```python
from build123d import *

# Parameters (mm, degrees)
SKETCH1_W           = 100
SKETCH1_H           = 100
BASE_DEPTH          = 10
SKETCH2_R           = 10.5
LOAD_CELL_CUT_DEPTH = 1
CUT_EXTRUDE1_REACH  = 12
SKETCH15_R          = 3
SKETCH21_R          = 2.5
CUT_EXTRUDE2_DEPTH  = 10
SKETCH22_R          = 4
CUT_EXTRUDE3_DEPTH  = 11


with BuildPart() as part:
    # Sketch1 → base (new body)
    with BuildSketch(Plane(origin=(0, 0, 0), x_dir=(1, 0, 0), z_dir=(0, 1, 0))):
        Rectangle(SKETCH1_W, SKETCH1_H)
    extrude(amount=BASE_DEPTH)

    # Sketch2 → load cell cut (cut)
    with BuildSketch(Plane(origin=(0, 10, 0), x_dir=(1, 0, 0), z_dir=(0, 1, 0))):
        Circle(SKETCH2_R)
    extrude(amount=-LOAD_CELL_CUT_DEPTH, mode=Mode.SUBTRACT)

    # Sketch15 → Cut-Extrude1 (cut, up to next)
    with BuildSketch(Plane(origin=(0, 0, 0), x_dir=(-1, 0, 0), z_dir=(0, -1, 0)), mode=Mode.PRIVATE) as cut_extrude1_sk1:
        with Locations((40, -40)):
            Circle(SKETCH15_R)
    cut_extrude1_tool1 = extrude(cut_extrude1_sk1.sketch, amount=-CUT_EXTRUDE1_REACH, mode=Mode.PRIVATE) & part.part
    add(cut_extrude1_tool1.solids().sort_by_distance((-40, 0, 40))[0], mode=Mode.SUBTRACT)
    # Sketch15 → Cut-Extrude1 (cut, up to next)
    with BuildSketch(Plane(origin=(0, 0, 0), x_dir=(-1, 0, 0), z_dir=(0, -1, 0)), mode=Mode.PRIVATE) as cut_extrude1_sk2:
        with Locations((-40, -40)):
            Circle(SKETCH15_R)
    cut_extrude1_tool2 = extrude(cut_extrude1_sk2.sketch, amount=-CUT_EXTRUDE1_REACH, mode=Mode.PRIVATE) & part.part
    add(cut_extrude1_tool2.solids().sort_by_distance((40, 0, 40))[0], mode=Mode.SUBTRACT)
    # Sketch15 → Cut-Extrude1 (cut, up to next)
    with BuildSketch(Plane(origin=(0, 0, 0), x_dir=(-1, 0, 0), z_dir=(0, -1, 0)), mode=Mode.PRIVATE) as cut_extrude1_sk3:
        with Locations((40, 40)):
            Circle(SKETCH15_R)
    cut_extrude1_tool3 = extrude(cut_extrude1_sk3.sketch, amount=-CUT_EXTRUDE1_REACH, mode=Mode.PRIVATE) & part.part
    add(cut_extrude1_tool3.solids().sort_by_distance((-40, 0, -40))[0], mode=Mode.SUBTRACT)
    # Sketch15 → Cut-Extrude1 (cut, up to next)
    with BuildSketch(Plane(origin=(0, 0, 0), x_dir=(-1, 0, 0), z_dir=(0, -1, 0)), mode=Mode.PRIVATE) as cut_extrude1_sk4:
        with Locations((-40, 40)):
            Circle(SKETCH15_R)
    cut_extrude1_tool4 = extrude(cut_extrude1_sk4.sketch, amount=-CUT_EXTRUDE1_REACH, mode=Mode.PRIVATE) & part.part
    add(cut_extrude1_tool4.solids().sort_by_distance((40, 0, -40))[0], mode=Mode.SUBTRACT)

    # Sketch21 → Cut-Extrude2 (cut)
    with BuildSketch(Plane(origin=(0, 0, -50), x_dir=(-1, 0, 0), z_dir=(0, 0, -1))):
        with Locations((-10, 5)):
            Circle(SKETCH21_R)
        with Locations((10, 5)):
            Circle(SKETCH21_R)
    cut_extrude2 = extrude(amount=-CUT_EXTRUDE2_DEPTH, mode=Mode.SUBTRACT)

    # Mirror2: Cut-Extrude2 across plane
    add(cut_extrude2.mirror(Plane.XY), mode=Mode.SUBTRACT)

    # Sketch22 → Cut-Extrude3 (cut, through all)
    with BuildSketch(Plane(origin=(0, 10, 0), x_dir=(1, 0, 0), z_dir=(0, 1, 0))):
        with Locations((40, -40)):
            Circle(SKETCH22_R)
        with Locations((-40, -40)):
            Circle(SKETCH22_R)
        with Locations((-40, 40)):
            Circle(SKETCH22_R)
        with Locations((40, 40)):
            Circle(SKETCH22_R)
    extrude(amount=-CUT_EXTRUDE3_DEPTH, mode=Mode.SUBTRACT)


solid = part.part
```
The listing builds one solid part. Answer for the finished solid, in the listing's coordinates (mm). A direction names the side the tool comes from. Give positions to 0.01 mm unless a question says otherwise; leave off trailing zeros. Order: outer loops, then holes, each group sorted by start corner. A loop starts at its lowest first (then second) coordinate and runs counter-clockwise, first axis right, second up. Notation, with made-up numbers: (-0.5, 8.5) -> (24.5, 8.5) arc R6 cw to (24.5, 19.5) -> close; hole circle Ø9 at (12.5, 78.25). An arc over 180 degrees is marked (long way). Answer as a JSON object with one key per item and string values. Group by question number.
Item 1: The part is cut by section D-D on x = 0. Write down the section's boundary in (y, z), and give its area (3 significant figures).
Item 2: The part is cut by section A-A on z = -42.5. Write down the section's boundary in (x, y).
Item 3: Flat-ended cylindrical pins translate along their axes: pin 1 (2.5 mm diameter, centred on x = -9, y = 4, fed in from -Z); pin 2 (3 mm diameter, centred on x = 10, y = 5, fed in from +Z); pin 3 (6.5 mm diameter, centred on x = 1, z = 2, fed in from +Y). Find the tip coordinate at first contact, or state that the pin passes through.
Item 4: Determine the mould class of faces 1 (the flat face through (-1, 10, -12)), 2 (the flat face through (0, 9, 0)), 3 (the flat face through (-1, 5, -50)) for opening direction Z: pulls with the +Z half, pulls with the -Z half, needs draft (parallel to the pull), parting line crosses it, or undercut.
Item 5: The part is cut by section C-C on z = 0. Write down the section's boundary in (x, y).
Item 6: The part is cut by section B-B on x = -40. Write down the section's boundary in (y, z), and give its area (3 significant figures).
Item 7: A tool of negligible diameter and unlimited length cuts with its end or side. For faces 4 (the flat face through (-10, 5, -40)), 5 (the cylindrical face through (10, 9.5, -3.2)), 6 (the flat face through (-10, 5, 40)), 7 (the flat face through (50, 5, 1)), 8 (the cylindrical face through (-40.521, 5.07, 36.034)), from which of +Z, -Z, +X, -X, +Y, -Y can it reach the whole face along a straight path? Write none if from no direction.
Item 8: Consider L1, parallel to Z at x = -40, y = 3.5; L2, parallel to Y at x = -10, z = 45.5; L3, parallel to X at y = 2.5, z = 38. Determine where each line is inside the solid, lowest interval first. Write a range as from..to.
Result set:
{
 "1": {"outline": "(0, -50) -> (10, -50) -> (10, -10.5) -> (9, -10.5) -> (9, 10.5) -> (10, 10.5) -> (10, 50) -> (0, 50) -> close", "area": "979 mm²"},
 "2": {"outline": "(-50, 0) -> (-43.12, 0) -> (-43.12, 10) -> (-50, 10) -> close; (-36.88, 0) -> (36.88, 0) -> (36.88, 10) -> (-36.88, 10) -> close; (43.12, 0) -> (50, 0) -> (50, 10) -> (43.12, 10) -> close; hole circle Ø5 at (-10, 5); hole circle Ø5 at (10, 5)"},
 "3": {"pin 1": "z = -50", "pin 2": "z = 40", "pin 3": "y = 9"},
 "4": {"face 1": "needs draft", "face 2": "undercut", "face 3": "pulls with the -Z half"},
 "5": {"outline": "(-50, 0) -> (50, 0) -> (50, 10) -> (10.5, 10) -> (10.5, 9) -> (-10.5, 9) -> (-10.5, 10) -> (-50, 10) -> close"},
 "6": {"outline": "(0, -50) -> (10, -50) -> (10, -44) -> (0, -44) -> close; (0, -36) -> (10, -36) -> (10, 36) -> (0, 36) -> close; (0, 44) -> (10, 44) -> (10, 50) -> (0, 50) -> close", "area": "840 mm²"},
 "7": {"face 4": "-Z", "face 5": "+Y", "face 6": "+Z", "face 7": "+Z, -Z, +X, +Y, -Y", "face 8": "+Y, -Y"},
 "8": {"L1": "-50..-44, -36..36, 44..50", "L2": "0..2.5, 7.5..10", "L3": "-50..-43.46, -36.54..36.54, 43.46..50"}
}
